Geometry check sheet. Reference: drawing and pictorial views, mm from the part's lowest x, y, z. A direction names the side the tool comes from. Round coordinates to 2 decimals unless told otherwise and drop trailing zeros. Loops run counter-clockwise (first coordinate to the right, second up) from the corner with the lowest first, then second, coordinate; pieces in that order, holes last. Notation, with made-up numbers: (-15.75, 41.25) - (19.25, 41.25) arc R21 ccw to (19.25, 56.25) - close; hole circle Ø9 at (22.5, 88). An arc over 180 degrees is marked (long way). Return JSON: item names as keys, results as strings.
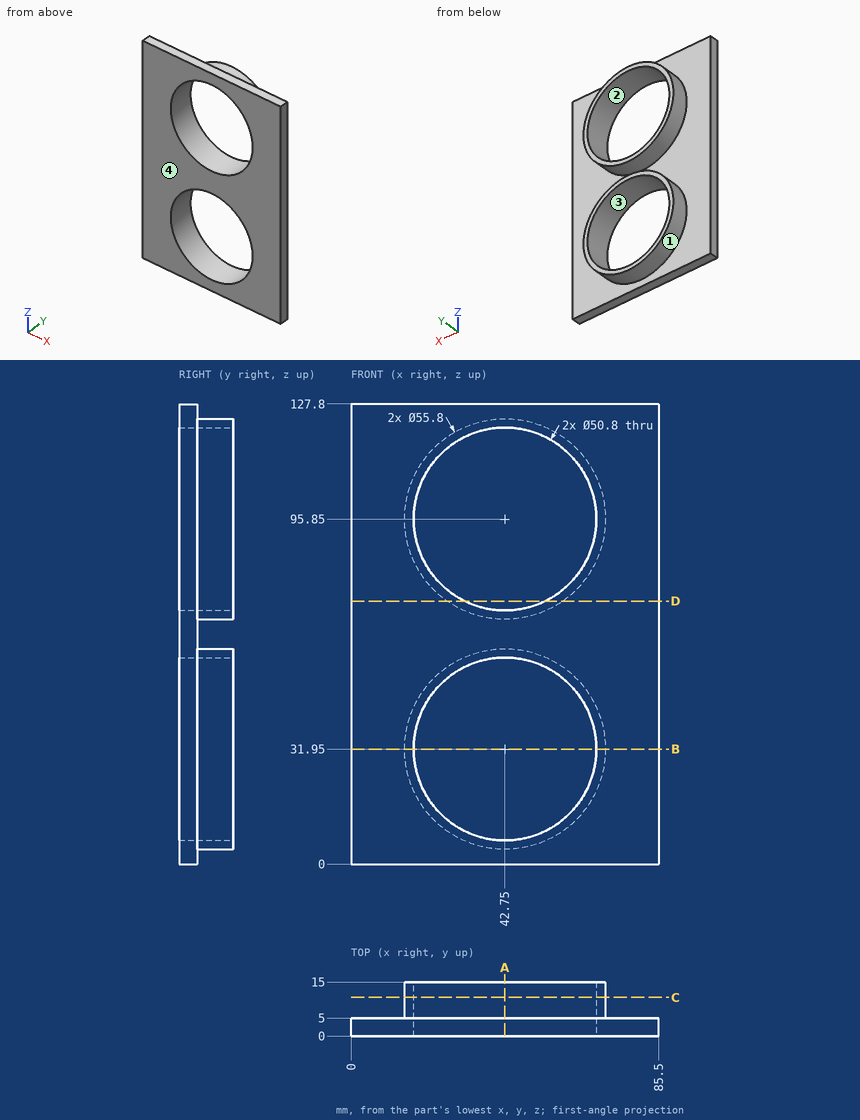
Q1. Sectioned sample at B-B (z = 31.95). Enter the section's corners in (x, y).
Answer key:
{"outline": "(0, 0) - (17.35, 0) - (17.35, 15) - (14.85, 15) - (14.85, 5) - (0, 5) - close; (68.15, 0) - (85.5, 0) - (85.5, 5) - (70.65, 5) - (70.65, 15) - (68.15, 15) - close"}
Q2. Sectioned sample at D-D (z = 73). Enter the section's corners in (x, y).
Answer key:
{"outline": "(0, 0) - (31.66, 0) - (31.66, 15) - (26.74, 15) - (26.74, 5) - (0, 5) - close; (53.84, 0) - (85.5, 0) - (85.5, 5) - (58.76, 5) - (58.76, 15) - (53.84, 15) - close"}
Q3. Sectioned sample at A-A (x = 42.75). Enter the section's corners in (y, z), plus the area to 3 significant figures.
Answer key:
{"outline": "(0, 0) - (5, 0) - (5, 4.05) - (15, 4.05) - (15, 6.55) - (0, 6.55) - close; (0, 57.35) - (15, 57.35) - (15, 59.85) - (5, 59.85) - (5, 67.95) - (15, 67.95) - (15, 70.45) - (0, 70.45) - close; (0, 121.25) - (15, 121.25) - (15, 123.75) - (5, 123.75) - (5, 127.8) - (0, 127.8) - close", "area": "231 mm²"}
Q4. Sectioned sample at C-C (y = 10.75). Enter the section's corners in (x, z), plus the area to 3 significant figures.
Answer key:
{"outline": "circle Ø55.8 at (42.75, 31.95); circle Ø55.8 at (42.75, 95.85); hole circle Ø50.8 at (42.75, 31.95); hole circle Ø50.8 at (42.75, 95.85)", "area": "837 mm²"}
Q5. Draft check along Z on the marked faces 3 and 4. Enter one of: released by +Z, released by -Z, zero draft, split by the parting line, or undercut.
Answer key:
{"face 3": "undercut", "face 4": "zero draft"}
Q6. Scan lines: probe 1 along Z at (x, y) = (42.75, 4); probe 2 along Z at (x, y) = (42.75, 7.75); probe 3 along Z at (x, y) = (33, 4.75). Record each from-to range of solid material in increasing order. Write a range as [from, to].
Answer key:
{"probe 1": "z = [0, 6.55], [57.35, 70.45], [121.25, 127.8]", "probe 2": "z = [4.05, 6.55], [57.35, 59.85], [67.95, 70.45], [121.25, 123.75]", "probe 3": "z = [0, 8.5], [55.4, 72.4], [119.3, 127.8]"}
Q7. Depth check by flat-ended pin: P1, Ø6, axis at y = 2, z = 73.5, coming from the -X side; P2, Ø4, axis at x = 26, y = 12.5, coming from the -Z side; P3, Ø3, axis at y = 11.5, z = 78.5, coming from the +X side; P4, Ø3, axis at y = 7.5, z = 76, coming from the -X side. Enter the tip coordinate at first touch or a pass-through.
Answer key:
{"P1": "stops at x = 0", "P2": "stops at z = 8.27", "P3": "stops at x = 65.71", "P4": "stops at x = 21.73"}
Q8. Tool access check on the marked faces 1 and 2. Record the directions out of +Z, -Z, +X, -X, +Y, -Y that give a thin tool (end or side, any length) a straight path to the whole face; none if there is none.
Answer key:
{"face 1": "+Y", "face 2": "+Y, -Y"}
